from build123d import *

# Parameters (mm, degrees)
SKETCH1_W                = 20
SKETCH1_H                = 70
SKETCH1_R                = 2.5
SKETCH1_W_2              = 57
SKETCH1_W_3              = 3
BOSS_EXTRUDE1_DEPTH      = 3
SKETCH1_3_W              = 3
SKETCH1_3_H              = 70
BOSS_EXTRUDE2_DEPTH      = 26
SKETCH2_R                = 2.5
CUT_EXTRUDE1_DEPTH       = 17
SKETCH3_R                = 1.5
SKETCH3_R_2              = 11.025
CUT_EXTRUDE2_DEPTH       = 10
FILLET1_R                = 20
BOSS_EXTRUDE4_START      = 26
SKETCH1_4_W              = 20
SKETCH1_4_H              = 70
SKETCH1_4_R              = 2.5
BOSS_EXTRUDE4_DEPTH      = 3
SKETCH4_R                = 6.5
SKETCH4_R_2              = 4
BOSS_EXTRUDE5_DEPTH      = 10
FILLET2_R                = 1
FILLET3_R                = 2
M5_CLEARANCE_HOLE1_D     = 5.5
M5_CLEARANCE_HOLE1_DEPTH = 23
M5_CLEARANCE_HOLE2_D     = 5.5


with BuildPart() as part:
    # Sketch1 → Boss-Extrude1 (new body)
    with BuildSketch(Plane(origin=(0, 0, 0), x_dir=(1, 0, 0), z_dir=(0, 1, 0))):
        with Locations((-30, 0)):
            Rectangle(SKETCH1_W, SKETCH1_H)
        with Locations((-30, -17.5)):
            Circle(SKETCH1_R, mode=Mode.SUBTRACT)
        with Locations((-30, 17.5)):
            Circle(SKETCH1_R, mode=Mode.SUBTRACT)
        with Locations((11.5, 0)):
            Rectangle(SKETCH1_W_2, SKETCH1_H)
        with Locations((-18.5, 0)):
            Rectangle(SKETCH1_W_3, SKETCH1_H)
    extrude(amount=BOSS_EXTRUDE1_DEPTH)

    # Sketch1<3> → Boss-Extrude2 (add)
    with BuildSketch(Plane(origin=(0, 0, 0), x_dir=(1, 0, 0), z_dir=(0, 1, 0))):
        with Locations((-18.5, 0)):
            Rectangle(SKETCH1_3_W, SKETCH1_3_H)
    extrude(amount=BOSS_EXTRUDE2_DEPTH)

    # Sketch2 → Cut-Extrude1 (cut)
    with BuildSketch(Plane(origin=(-17, 0, 0), x_dir=(0, 0, -1), z_dir=(1, 0, 0))):
        with Locations((-17.5, 13)):
            Circle(SKETCH2_R)
        with Locations((17.5, 13)):
            Circle(SKETCH2_R)
    extrude(amount=-CUT_EXTRUDE1_DEPTH, mode=Mode.SUBTRACT)

    # Sketch3 → Cut-Extrude2 (cut)
    with BuildSketch(Plane(origin=(0, 3, 0), x_dir=(1, 0, 0), z_dir=(0, 1, 0))):
        with Locations((-1.350000521, 15.500000521)):
            Circle(SKETCH3_R)
        with Locations((14.15, 0)):
            Circle(SKETCH3_R_2)
        with Locations((29.649999479, 15.499999479)):
            Circle(SKETCH3_R)
        with Locations((29.650000521, -15.500000521)):
            Circle(SKETCH3_R)
        with Locations((-1.349999479, -15.499999479)):
            Circle(SKETCH3_R)
    extrude(amount=-CUT_EXTRUDE2_DEPTH, mode=Mode.SUBTRACT)

    # Fillet1
    fillet1_edges = [part.edges().sort_by_distance(p)[0] for p in [
        (40, 1.5, -35),
        (40, 1.5, 35),
    ]]
    fillet(fillet1_edges, radius=FILLET1_R)

    # Sketch1<4> → Boss-Extrude4 (add)
    with BuildSketch(Plane(origin=(0, 0, 0), x_dir=(1, 0, 0), z_dir=(0, 1, 0)).offset(BOSS_EXTRUDE4_START)):
        with Locations((-30, 0)):
            Rectangle(SKETCH1_4_W, SKETCH1_4_H)
        with Locations((-30, -17.5)):
            Circle(SKETCH1_4_R, mode=Mode.SUBTRACT)
        with Locations((-30, 17.5)):
            Circle(SKETCH1_4_R, mode=Mode.SUBTRACT)
    extrude(amount=-BOSS_EXTRUDE4_DEPTH)

    # Sketch4 → Boss-Extrude5 (add)
    with BuildSketch(Plane(origin=(0, 3, 0), x_dir=(1, 0, 0), z_dir=(0, 1, 0))):
        with Locations((14.15, 22)):
            Circle(SKETCH4_R)
        with Locations((14.15, 22)):
            Circle(SKETCH4_R_2, mode=Mode.SUBTRACT)
    extrude(amount=BOSS_EXTRUDE5_DEPTH)

    # Fillet2
    fillet2_edges = [part.edges().sort_by_distance(p)[0] for p in [
        (-17, 14.5, -35),
        (-17, 14.5, 35),
        (1.5, 3, -35),
        (34.142135624, 3, -29.142135624),
        (40, 3, 0),
        (34.142135624, 3, 29.142135624),
        (-17, 3, 0),
        (-17, 26, 0),
        (1.5, 3, 35),
        (-20, 3, 0),
        (-40, 23, 0),
        (-40, 3, 0),
        (-40, 26, 0),
    ]]
    fillet(fillet2_edges, radius=FILLET2_R)

    # Fillet3
    fillet3_edges = [part.edges().sort_by_distance(p)[0] for p in [
        (7.65, 13, -22),
        (7.65, 3, -22),
    ]]
    fillet(fillet3_edges, radius=FILLET3_R)

    # M5 Clearance Hole1
    with Locations(Plane(origin=(-17, 0, 0), x_dir=(0, 0, -1), z_dir=(1, 0, 0))):
        with Locations((-17.5, 13), (17.5, 13)):
            Hole(M5_CLEARANCE_HOLE1_D / 2, depth=M5_CLEARANCE_HOLE1_DEPTH)

    # M5 Clearance Hole2 (through all)
    with Locations(Plane(origin=(0, 26, 0), x_dir=(1, 0, 0), z_dir=(0, 1, 0))):
        with Locations((-30, -17.5), (-30, 17.5)):
            Hole(M5_CLEARANCE_HOLE2_D / 2)


solid = part.part
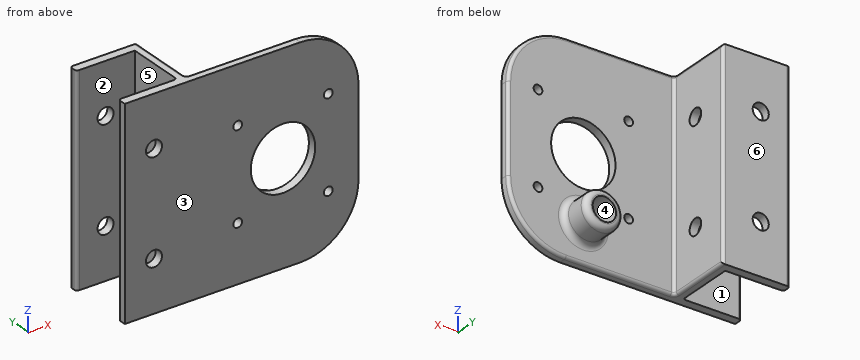
Geometry check sheet. Reference: the model listing, model coordinates, mm. Face numbers are marked on the shaded views. A direction names the side the tool comes from. Coordinates: 2 decimals unless noted, no trailing zeros. Order: outer loops, then holes, each group sorted by start corner. A loop starts at its lowest first (then second) coordinate and runs counter-clockwise, first axis right, second up. Notation, with made-up numbers: (-6, -27.5) - (-1, -27.5) arc R20 cw to (-1, -13.5) - close; hole circle Ø2 at (31, 47). An arc over 180 degrees is marked (long way). Answer in a Markdown table with one row per item. Add a question column.
1) Cross-section at C-C, the plane y = 20.5. Record the cut outline in (x, z).
2) Cross-section at A-A, the plane x = -30. Record the cut outline in (y, z), then the cut area to 3 significant figures.
3) Material ranges on line 1 along Z through (x, y) = (-30, 0.7); line 2 along X through (y, z) = (7.25, -22); line 3 along Y through (x, z) = (-36, 24.5), recorded low to high. Write a range as [from, to].
4) Release check for a two-part mould opening along Y. For the marked faces 1, 2, 3 and 4 record: +Y half, -Y half, draft (parallel to the pull), parting line (faces both ways), or undercut.
5) Cross-section at D-D, the plane z = -4.5. Record the cut outline in (x, y).
6) Set-up check for the marked faces 5 and 6: record each of +Z, -Z, +X, -X, +Y, -Y from which the full face is reachable in a straight line by a thin tool's end or side.
7) Gauge pin test, flat ends, axial feed: P1, Ø6.5, axis at x = 14.15, z = -22, coming from the -Y side; P2, Ø3, axis at x = 7.5, z = 14, coming from the +Y side; P3, Ø8, axis at y = 23, z = 25, coming from the +X side; P4, Ø6.5, axis at y = 13, z = -17.5, coming from the -X side. Record the tip position at first contact, or that the pin passes through.
8) Cross-section at B-B, the plane z = 7.5. Record the cut outline in (x, y).
Check result:
| question | item | result |
|---|---|---|
| 1 | outline | (-20, -35) - (-18, -35) arc R1 ccw to (-17, -34) - (-17, 34) arc R1 ccw to (-18, 35) - (-20, 35) - close |
| 2 | outline | (0, -35) - (3, -35) - (3, -20.25) - (0, -20.25) - close; (0, -14.75) - (3, -14.75) - (3, 14.75) - (0, 14.75) - close; (0, 20.25) - (3, 20.25) - (3, 35) - (0, 35) - close; (23, -35) - (26, -35) - (26, -20.25) - (23, -20.25) - close; (23, -14.75) - (26, -14.75) - (26, 14.75) - (23, 14.75) - close; (23, 20.25) - (26, 20.25) - (26, 35) - (23, 35) - close |
| 2 | area | 354 mm² |
| 3 | line 1 | z = [-35, -20.25], [-14.75, 14.75], [20.25, 35] |
| 3 | line 2 | x = [-20, -17], [7.65, 10.15], [18.15, 20.65] |
| 3 | line 3 | y = [0, 3], [23, 26] |
| 4 | face 1 | undercut |
| 4 | face 2 | undercut |
| 4 | face 3 | -Y half |
| 4 | face 4 | draft |
| 5 | outline | (-40, 0) - (4.09, 0) - (4.09, 3) - (-16, 3) arc R1 cw to (-17, 4) - (-17, 25) arc R1 ccw to (-18, 26) - (-39, 26) arc R1 ccw to (-40, 25) - (-40, 24) arc R1 ccw to (-39, 23) - (-20, 23) - (-20, 4) arc R1 cw to (-21, 3) - (-39, 3) arc R1 ccw to (-40, 2) - close; (24.21, 0) - (40, 0) - (40, 2) arc R1 ccw to (39, 3) - (24.21, 3) - close |
| 6 | face 5 | +Z, -Z, -X |
| 6 | face 6 | +Z, -Z, +X, -X, +Y |
| 7 | P1 | stops at y = 0 |
| 7 | P2 | stops at y = 3 |
| 7 | P3 | stops at x = -17 |
| 7 | P4 | stops at x = -20 |
| 8 | outline | (-40, 0) - (6.07, 0) - (6.07, 3) - (-16, 3) arc R1 cw to (-17, 4) - (-17, 25) arc R1 ccw to (-18, 26) - (-39, 26) arc R1 ccw to (-40, 25) - (-40, 24) arc R1 ccw to (-39, 23) - (-20, 23) - (-20, 4) arc R1 cw to (-21, 3) - (-39, 3) arc R1 ccw to (-40, 2) - close; (22.23, 0) - (40, 0) - (40, 2) arc R1 ccw to (39, 3) - (22.23, 3) - close |
